Autodesk Inventor part; units mm, degrees
ref_plane "YZ Plane" through (0, 0, 0) normal (1, 0, 0) x (0, 1, 0)
ref_plane "XZ Plane" through (0, 0, 0) normal (0, 1, 0) x (-1, 0, 0)
ref_plane "XY Plane" through (0, 0, 0) normal (0, 0, 1) x (1, 0, 0)
sketch "Sketch1" plane through (0, 0, 0) normal (1, 0, 0) x (0, 1, 0)
  line L0 (0, 21.9163) -> (-204, 21.9163)
  line L1 (-204, 21.9163) -> (-204, -13.7156)
  line L2 (-204, -13.7156) -> (0, -13.7156)
  line L3 (0, -13.7156) -> (0, 21.9163)
  line L4 (-4.9174, 21.9163) -> (-3, 0)
  line L5 (-3, 0) -> (-102.6195, -8.7156)
  line L6 (-102.6195, -8.7156) -> (-102.6195, -13.7156)
  line L7 (-102.6195, -13.7156) -> (0, -13.7156)
  point P0 (0, 0)
  dimension "d0" = 204
  dimension "d2" = 22
  dimension "d3" = 85
  dimension "d5" = 3
  dimension "d6" = 100
  dimension "d7" = 5
extrude "Extrusion1" add sketch "Sketch1" along normal mid plane 48.6667 contours L3 L2 L6 L5 L4 L0
properties part number "stand"
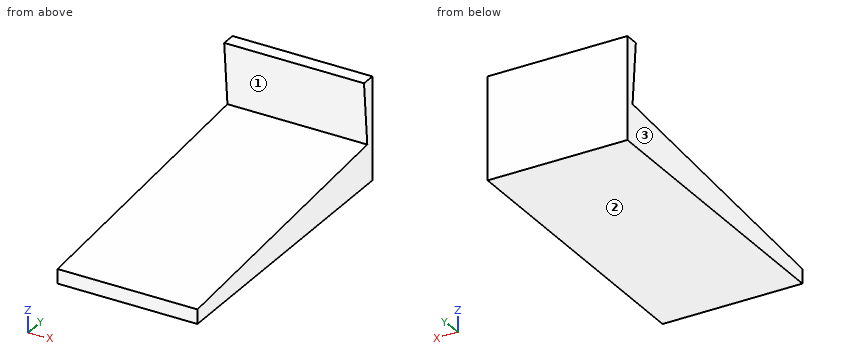
Could you check a few things on this model? Use its own coordinates, in mm. Face numbers are marked on the shaded views. Give positions to 0.01 mm unless a question says otherwise; leave off trailing zeros. Order: outer loops, then holes, each group sorted by start corner. A loop starts at its lowest first (then second) coordinate and runs counter-clockwise, first axis right, second up. Notation, with made-up numbers: (81, 17) - (99, 17) arc R28 ccw to (99, 45) - close; hole circle Ø10 at (-36.5, 52). An arc over 180 degrees is marked (long way). One line per item, written item: value. Start each with the question number.
1. Imagine slicing it at A-A on x = 15. List the corners of the cut face in (y, z) for me.
2. Thinking about a two-plate mould opening in Z: for the marked faces 1, 2 and 3, which applies, +Z half, -Z half, draft (parallel to the pull), parting line (faces both ways), or undercut?
3. Imagine slicing it at B-B on y = -66. List the corners of the cut face in (x, z) for me.
4. For P1, Ø12, axis at x = -18, y = -59.5, coming from the +Z side; P2, Ø4, axis at x = 12, z = 9.5, coming from the -Y side; P3, Ø6, axis at x = -9, z = 14.5, coming from the -Y side, each with a flat end and sliding along its axis, tell me the tip position at first contact or that it passes through.
5. If I drill on probe 1 along Y at (x, z) = (-15, 16); probe 2 along Y at (x, z) = (19, 0.5); probe 3 along Z at (x, y) = (-19, -83.5), over which ranges is the centre line in solid material (lowest first)?
6. Imagine slicing it at C-C on z = -7.5. List the corners of the cut face in (x, y) for me, plus the area to 3 significant figures.
Values:
1. outline: (-102.62, -13.72) - (0, -13.72) - (0, 21.92) - (-4.92, 21.92) - (-3, 0) - (-102.62, -8.72) - close
2. face 1: undercut
2. face 2: -Z half
2. face 3: draft
3. outline: (-24.33, -13.72) - (24.33, -13.72) - (24.33, -5.51) - (-24.33, -5.51) - close
4. P1: z = -4.42
4. P2: y = -4.01
4. P3: y = -4.53
5. probe 1: -4.4 to 0
5. probe 2: -3.04 to 0
5. probe 3: -13.72 to -7.04
6. outline: (-24.33, -88.73) - (24.33, -88.73) - (24.33, 0) - (-24.33, 0) - close
6. area: 4,320 mm²
